```python
from build123d import *

# Parameters (mm, degrees)
SZKIC4_W                        = 63
SZKIC4_H                        = 12.5
WYTNIJ_WYCI_GNI_CIE1_DEPTH      = 12.5
WYTNIJ_WYCI_GNI_CIE1_DEPTH_BACK = 12.5
SZKIC1_W                        = 4
SZKIC1_H                        = 16
WYTNIJ_WYCI_GNI_CIE2_DEPTH      = 12.5
WYTNIJ_WYCI_GNI_CIE2_DEPTH_BACK = 12.5
SZKIC2_W                        = 4
SZKIC2_H                        = 16


with BuildPart() as part:
    # Szkic3 → Obr_t1 (revolve)
    with BuildSketch(Plane(origin=(0, 0, 0), x_dir=(0, 0, -1), z_dir=(1, 0, 0)), mode=Mode.PRIVATE) as obr_t1_sk:
        Polygon((-25, 0), (-25, 8), (-1.227, 8), (0, 6.773), (0, 0), align=None)
    revolve(obr_t1_sk.sketch.rotate(Axis((0, 0, 0), (0, 0, 1)), 270), axis=Axis((0, 0, 0), (0, 0, 1)))

    # Szkic4 → Obr_t2 (revolve)
    with BuildSketch(Plane(origin=(0, 0, 0), x_dir=(0, 0, -1), z_dir=(1, 0, 0)), mode=Mode.PRIVATE) as obr_t2_sk:
        with Locations((-56.5, 6.25)):
            Rectangle(SZKIC4_W, SZKIC4_H)
    revolve(obr_t2_sk.sketch.rotate(Axis((0, 0, 25), (0, 0, 1)), 270), axis=Axis((0, 0, 25), (0, 0, 1)))

    # Szkic5 → Wyci_cie-obr_t1 (revolve, cut)
    with BuildSketch(Plane(origin=(0, 0, 0), x_dir=(0, 0, -1), z_dir=(1, 0, 0)), mode=Mode.PRIVATE) as wyci_cie_obr_t1_sk:
        Polygon((-88, 10.2372583), (-85.7372583, 12.5), (-88, 12.5), align=None)
    revolve(wyci_cie_obr_t1_sk.sketch.rotate(Axis((0, 0, 25), (0, 0, 1)), 270), axis=Axis((0, 0, 25), (0, 0, 1)), mode=Mode.SUBTRACT)

    # Szkic6 → Wyci_cie-obr_t2 (revolve, cut)
    with BuildSketch(Plane(origin=(0, 0, 0), x_dir=(0, 0, -1), z_dir=(1, 0, 0)), mode=Mode.PRIVATE) as wyci_cie_obr_t2_sk:
        with BuildLine():
            Line((-23.4, 8), (-25, 8))
            ThreePointArc((-25, 8), (-24.2, 7.2), (-23.4, 8))
        make_face()
    revolve(wyci_cie_obr_t2_sk.sketch.rotate(Axis((0, 0, 0), (0, 0, 1)), 270), axis=Axis((0, 0, 0), (0, 0, 1)), mode=Mode.SUBTRACT)

    # Szkic1 → Wytnij-wyci_gni_cie1 (cut, two sides: drawn at the far end of the back side and taken through both)
    with BuildSketch(Plane(origin=(0, 0, 0), x_dir=(1, 0, 0), z_dir=(0, 1, 0)).offset(-WYTNIJ_WYCI_GNI_CIE1_DEPTH_BACK)):
        with Locations((13, -48)):
            Rectangle(SZKIC1_W, SZKIC1_H)
    extrude(amount=WYTNIJ_WYCI_GNI_CIE1_DEPTH + WYTNIJ_WYCI_GNI_CIE1_DEPTH_BACK, mode=Mode.SUBTRACT)

    # Szkic2 → Wytnij-wyci_gni_cie2 (cut, two sides: drawn at the far end of the back side and taken through both)
    with BuildSketch(Plane(origin=(0, 0, 0), x_dir=(1, 0, 0), z_dir=(0, 1, 0)).offset(-WYTNIJ_WYCI_GNI_CIE2_DEPTH_BACK)):
        with Locations((-13, -48)):
            Rectangle(SZKIC2_W, SZKIC2_H)
    extrude(amount=WYTNIJ_WYCI_GNI_CIE2_DEPTH + WYTNIJ_WYCI_GNI_CIE2_DEPTH_BACK, mode=Mode.SUBTRACT)


solid = part.part
```
The model under review builds one solid part; all positions refer to its coordinate system, in mm. A direction names the side the tool comes from. Round coordinates to 2 decimals unless told otherwise and drop trailing zeros. Order: outer loops, then holes, each group sorted by start corner. A loop starts at its lowest first (then second) coordinate and runs counter-clockwise, first axis right, second up. Notation, with made-up numbers: (-30, 0.25) - (-6, 0.25) arc R16 cw to (-6, 13.25) - close; hole circle Ø1 at (-4.75, 43.5). An arc over 180 degrees is marked (long way). Answer in a Markdown table with one row per item.
(1) Take a section at D-D on z = 22. Write out the cut boundary in (x, y), plus the area to 3 significant figures.
Result set:
| item | result |
|---|---|
| outline | circle Ø16 at (0, 0) |
| area | 201 mm2 |
(2) Take a section at C-C on z = 53. Write out the cut boundary in (x, y).
Result set:
| item | result |
|---|---|
| outline | (-11, -5.94) arc R12.5 ccw to (11, -5.94) - (11, 5.94) arc R12.5 ccw to (-11, 5.94) - close |
(3) Take a section at A-A on y = 0. Write out the cut boundary in (x, z), plus the area to 3 significant figures.
Result set:
| item | result |
|---|---|
| outline | (-12.5, 25) - (-8, 25) arc R0.8 cw to (-8, 23.4) - (-8, 1.23) - (-6.77, 0) - (6.77, 0) - (8, 1.23) - (8, 23.4) arc R0.8 cw to (8, 25) - (12.5, 25) - (12.5, 40) - (11, 40) - (11, 56) - (12.5, 56) - (12.5, 85.74) - (10.24, 88) - (-10.24, 88) - (-12.5, 85.74) - (-12.5, 56) - (-11, 56) - (-11, 40) - (-12.5, 40) - close |
| area | 1,920 mm2 |
(4) Take a section at B-B on x = 0. Write out the cut boundary in (y, z), plus the area to 3 significant figures.
Result set:
| item | result |
|---|---|
| outline | (-12.5, 25) - (-8, 25) arc R0.8 cw to (-8, 23.4) - (-8, 1.23) - (-6.77, 0) - (6.77, 0) - (8, 1.23) - (8, 23.4) arc R0.8 cw to (8, 25) - (12.5, 25) - (12.5, 85.74) - (10.24, 88) - (-10.24, 88) - (-12.5, 85.74) - close |
| area | 1,970 mm2 |
(5) Machinability: for faces 1 (the face through (0.2, -8.2, 25)), 2 (the face through (-12, 0, 56)), 3 (the face through (-2.25, -10.13, 87.86)), 4 (the face through (12, 0, 40)), which of the approach directions +Z, -Z, +X, -X, +Y, -Y give a long, thin tool a straight path to every point of the face, cutting with its end or side? Answer none if there is none.
Result set:
| item | result |
|---|---|
| face 1 | -Z |
| face 2 | -X, +Y, -Y |
| face 3 | +Z |
| face 4 | +X, +Y, -Y |
(6) Clearance check with flat-ended pins moving along their axes: P1, Ø2, axis at y = -3, z = 28.5, coming from the -X side; P2, Ø1, axis at x = 6, y = 10, coming from the -Z side; P3, Ø13, axis at y = 2.5, z = 44, coming from the -X side; P4, Ø1.5, axis at y = 4, z = 67.5, coming from the -X side. State where each tip first meets the part, or that it passes through.
Result set:
| item | result |
|---|---|
| P1 | stops at x = -12.34 |
| P2 | stops at z = 25 |
| P3 | stops at x = -12.5 |
| P4 | stops at x = -12.07 |
(7) Mouldability with a two-part tool opening along Z and no side actions: class faces 5 (the face through (-11, 0, 48)), 6 (the face through (0, 0, 0)), 7 (the face through (-1.73, -7.81, 12.16)) as released by +Z, released by -Z, zero draft, split by the parting line, or undercut.
Result set:
| item | result |
|---|---|
| face 5 | undercut |
| face 6 | released by -Z |
| face 7 | zero draft |
(8) For line 1 (X direction, y = -2.25, z = 53); line 2 (Z direction, x = -3.5, y = 8); line 3 (Z direction, x = -0.5, y = 7.5), list the stretches that pass through material, from the lowest coordinate up. Write a range as from..to.
Result set:
| item | result |
|---|---|
| line 1 | x = -11..11 |
| line 2 | z = 25..88 |
| line 3 | z = 0.74..23.56, 24.84..88 |
